Could you check a few things on this model? Use its own coordinates, in mm. Face numbers are marked on the shaded views. Coordinates: 2 decimals unless noted, no trailing zeros. Loops run counter-clockwise (first coordinate to the right, second up) from the corner with the lowest first, then second, coordinate; pieces in that order, holes last.
1) Imagine slicing it at D-D on x = 51. Please give me the cut outline in (y, z), plus the area to 3 significant figures.
2) Imagine slicing it at B-B on z = 84. Please give me the cut outline in (x, y), plus the area to 3 significant figures.
3) If I drill on line 1 along Y through (x, z) = (34.5, 102.5); line 2 along X through (y, z) = (10.75, 13); line 3 along Z through (x, y) = (96, 3.25), over which ranges is the centre line in solid material (lowest first)?
4) Imagine slicing it at A-A on x = 120. Please give me the cut outline in (y, z), plus the area to 3 significant figures.
5) Imagine slicing it at C-C on z = 46. Please give me the cut outline in (x, y), plus the area to 3 significant figures.
6) Will this pin go through, and if not, where does the flat tip stop? P1, Ø18, axis at x = 28.24, z = 40.04, coming from the -Y side.
7) Thinking about a two-plate mould opening in X: for the marked faces 1, 2 and 3, which applies, released by +X, released by -X, zero draft, split by the parting line, or undercut?
```python
from build123d import *

# Parameters (mm, degrees)
SKETCH_1_W          = 180
SKETCH_1_H          = 120
EXTRUDE_2_DEPTH     = 30
SKETCH_3_R          = 30
SKETCH_3_R_2        = 11.186038902
CUT_EXTRUDE_1_DEPTH = 213.807433918
FILLET_1_R          = 20
SHELL_1_T           = 2


with BuildPart() as part:
    # 草图1 → 凸台-拉伸2 (new body)
    with BuildSketch(Plane(origin=(0, 0, 0), x_dir=(1, 0, 0), z_dir=(0, 1, 0))):
        with Locations((90, -49.485176763)):
            Rectangle(SKETCH_1_W, SKETCH_1_H)
    extrude(amount=EXTRUDE_2_DEPTH)

    # 草图3 → 切除-拉伸1 (cut, through all)
    with BuildSketch(Plane(origin=(0, 30, 0), x_dir=(1, 0, 0), z_dir=(0, 1, 0))):
        with Locations(Location((120, -57.523652535, 0), (0, 0, 270))):
            Circle(SKETCH_3_R)
        with Locations(Location((28.239340808, -40.043809648, 0), (0, 0, 270))):
            Circle(SKETCH_3_R_2)
    extrude(amount=-CUT_EXTRUDE_1_DEPTH, mode=Mode.SUBTRACT)

    # 圆角1
    fillet_1_edges = [part.edges().sort_by_distance(p)[0] for p in [
        (0, 15, -10.514823237),
        (180, 15, -10.514823237),
        (180, 15, 109.485176763),
        (0, 15, 109.485176763),
    ]]
    fillet(fillet_1_edges, radius=FILLET_1_R)

    # 抽壳1 (no face opened: a closed hollow body)
    add(offset(amount=-SHELL_1_T, mode=Mode.PRIVATE), mode=Mode.SUBTRACT)


solid = part.part
```
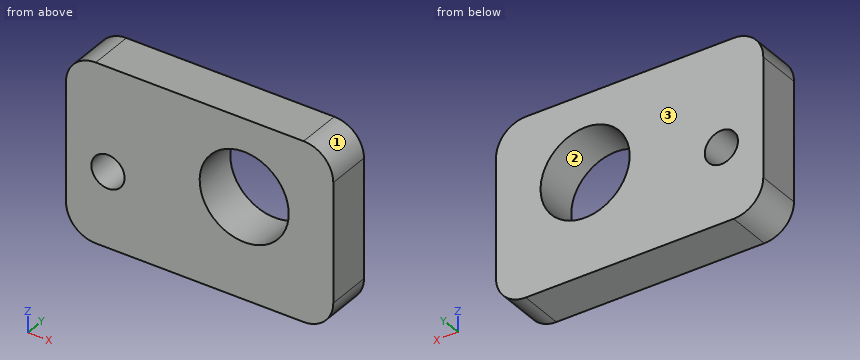
Filled in:
1. outline: (0, -10.51) - (30, -10.51) - (30, 109.49) - (0, 109.49) - close; hole (2, -8.51) - (28, -8.51) - (28, 107.49) - (2, 107.49) - close
1. area: 584 mm2
2. outline: (0, 0) - (105.89, 0) - (105.89, 30) - (0, 30) - close; (134.11, 0) - (180, 0) - (180, 30) - (134.11, 30) - close; hole (2, 2) - (102.03, 2) - (102.03, 28) - (2, 28) - close; hole (137.97, 2) - (178, 2) - (178, 28) - (137.97, 28) - close
2. area: 912 mm2
3. line 1: y = 0 to 2, 28 to 30
3. line 2: x = 0 to 2, 178 to 180
3. line 3: z = -10.51 to -8.51, 36.36 to 39.52, 75.52 to 78.69, 107.49 to 109.49
4. outline: (0, -10.51) - (30, -10.51) - (30, 27.52) - (0, 27.52) - close; (0, 87.52) - (30, 87.52) - (30, 109.49) - (0, 109.49) - close; hole (2, -8.51) - (28, -8.51) - (28, 25.52) - (2, 25.52) - close; hole (2, 89.52) - (28, 89.52) - (28, 107.49) - (2, 107.49) - close
4. area: 448 mm2
5. outline: (0, 0) - (18.77, 0) - (18.77, 30) - (0, 30) - close; (37.71, 0) - (92.3, 0) - (92.3, 30) - (37.71, 30) - close; (147.7, 0) - (180, 0) - (180, 30) - (147.7, 30) - close; hole (2, 2) - (16.48, 2) - (16.48, 28) - (2, 28) - close; hole (40, 2) - (90.15, 2) - (90.15, 28) - (40, 28) - close; hole (149.85, 2) - (178, 2) - (178, 28) - (149.85, 28) - close
5. area: 758 mm2
6. P1: passes through
7. face 1: released by +X
7. face 2: undercut
7. face 3: zero draft
